Here's how the part is built. I have some questions about the finished solid (model axes, mm). Give positions to 0.01 mm unless a question says otherwise; leave off trailing zeros. Order: outer loops, then holes, each group sorted by start corner. A loop starts at its lowest first (then second) coordinate and runs counter-clockwise, first axis right, second up. Notation, with made-up numbers: M 55.5,43 L 92.5,43 A24 ccw 92.5,62 Z; hole C -11,-33 d8. An arc over 180 degrees is marked long. One line per item, written item: value. Start each with the question number.
from build123d import *

# Parameters (mm, degrees)
SKETCH1_R                = 50.8
BOSS_EXTRUDE1_DEPTH      = 12.7
SKETCH2_R                = 6.35
BOSS_EXTRUDE2_DEPTH      = 114.3
BOSS_EXTRUDE2_DEPTH_BACK = 35.56
SKETCH4_R                = 6.35


with BuildPart() as part:
    # Sketch1 → Boss-Extrude1 (new body)
    with BuildSketch(Plane.XY):
        Circle(SKETCH1_R)
    extrude(amount=BOSS_EXTRUDE1_DEPTH)

    # Sketch2 → Boss-Extrude2 (add, two sides)
    with BuildSketch(Plane(origin=(0, 0, 0), x_dir=(-1, 0, 0), z_dir=(0, 0, -1))) as boss_extrude2_sk:
        Circle(SKETCH2_R)
    extrude(amount=BOSS_EXTRUDE2_DEPTH)
    extrude(boss_extrude2_sk.sketch, amount=-BOSS_EXTRUDE2_DEPTH_BACK)

    # Sweep3: sweep along a path in Sketch3
    with BuildLine(Plane(origin=(0, 0, 0), x_dir=(1, 0, 0), z_dir=(0, 1, 0))) as sweep3_path:
        ThreePointArc((0, -66.04), (15.24, -50.8), (0, -35.56))
    # Sketch4 → Sweep3 (sweep)
    with BuildSketch(Plane.XY.offset(50.8)):
        with Locations((15.298746374, 0)):
            Circle(SKETCH4_R)
    sweep3 = sweep(path=sweep3_path.line)

    # Mirror1: Sweep3 across plane
    add(sweep3.mirror(Plane(origin=(0, 0, 66.098746374), x_dir=(0, 0, 1), z_dir=(-1, 0, 0))))


solid = part.part
Item 1: Please list where these lines run through material, in increasing order: probe 1 along Z at (x, y) = (7.5, 4); probe 2 along Z at (x, y) = (23.5, 1); probe 3 along Z at (x, y) = (-13, -2). Write a range as [from, to].
Item 2: I want a section at D-D on x = -34. Write out the boundary of the cut face in (y, z), plus the area to 3 significant figures.
Item 3: I want a section at A-A on y = 0. Write out the boundary of the cut face in (x, z).
Item 4: I want a section at C-C on y = 20.5. Write out the boundary of the cut face in (x, z), plus the area to 3 significant figures.
Item 5: We'd pull the mould along Z, two halves only. Please class faces 1 (the face through (1.38, -6.2, -56.35)), 2 (the face through (-6.057, 1.907, 21.408)), 3 (the face through (0, 0, -114.3)): +Z half, -Z half, draft (parallel to the pull), parting line (faces both ways), or undercut.
Item 6: Will these pins go through, and if not, where does the flat tip stop? P1, Ø10, axis at y = 4, z = 41.5, coming from the +X side; P2, Ø6, axis at x = 18, z = 3, coming from the +Y side; P3, Ø2, axis at x = 4, y = -9, coming from the +Z side.
Item 7: I want a section at B-B on z = -62. Write out the boundary of the cut face in (x, y).
Answer below:
1. probe 1: z = [0, 12.7], [32.01, 43.64], [57.96, 69.59]
1. probe 2: z = [0, 12.7]
1. probe 3: z = [0, 12.7], [33.89, 67.71]
2. outline: M -37.74,0 L 37.74,0 L 37.74,12.7 L -37.74,12.7 Z
2. area: 959 mm²
3. outline: M -50.8,0 L -6.35,0 L -6.35,-114.3 L 6.35,-114.3 L 6.35,0 L 50.8,0 L 50.8,12.7 L 6.35,12.7 L 6.35,30.1 A21.65 ccw long -6.35,30.1 L -6.35,12.7 L -50.8,12.7 Z; hole C 0,50.8 d17.9
4. outline: M -46.48,0 L 46.48,0 L 46.48,12.7 L -46.48,12.7 Z
4. area: 1,180 mm²
5. face 1: draft
5. face 2: undercut
5. face 3: -Z half
6. P1: stops at x = 20.91
6. P2: stops at y = 48.53
6. P3: stops at z = 12.7
7. outline: C 0,0 d12.7
